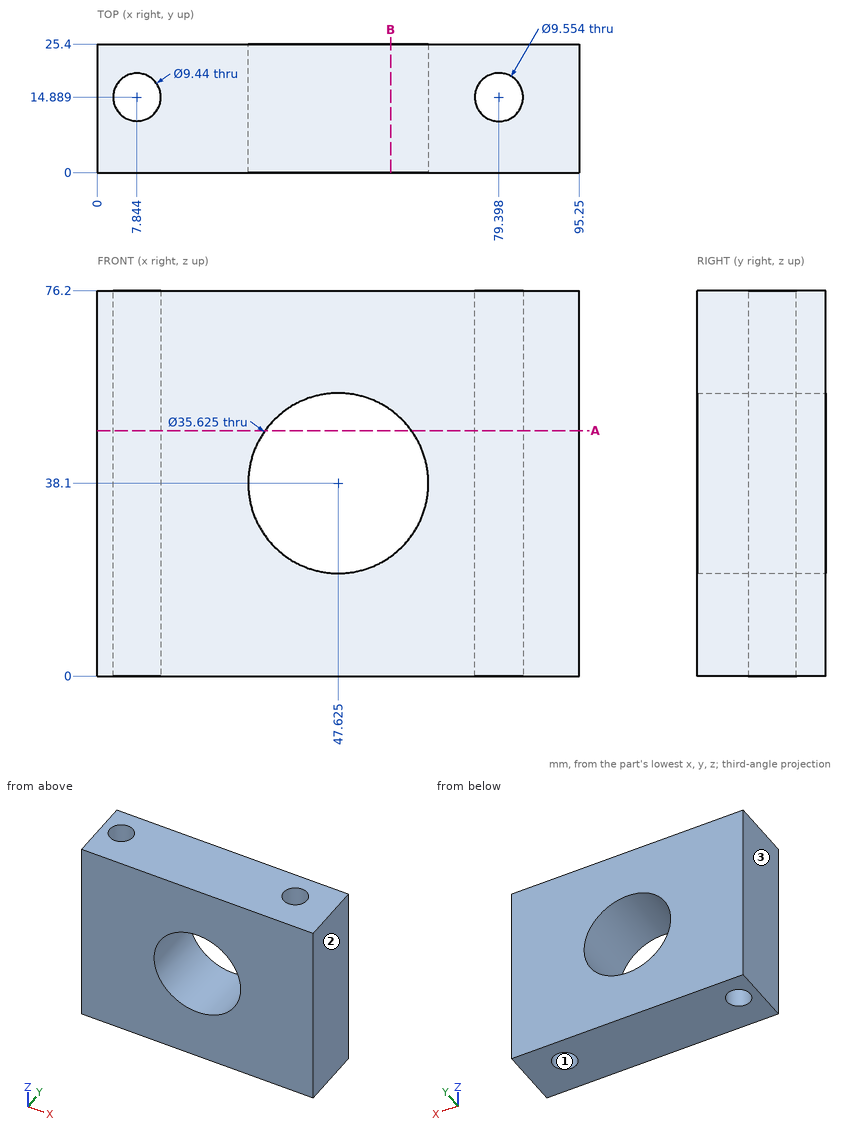
For this review, use the dimensioned drawing (mm, ordinates from the lowest corner) and the shaded views. Round coordinates to 2 decimals unless told otherwise and drop trailing zeros. Order: outer loops, then holes, each group sorted by start corner. A loop starts at its lowest first (then second) coordinate and runs counter-clockwise, first axis right, second up. Notation, with made-up numbers: (-5.5, 87) -> (45.5, 87) arc R33 ccw to (45.5, 120) -> close; hole circle Ø3 at (87.25, 34.5). An arc over 180 degrees is marked (long way). Write item = value, one per line. Start each with the question number.
Item 1: For line 1 along Z through (x, y) = (47, 14.5); line 2 along X through (y, z) = (3, 39.5); line 3 along Y through (x, z) = (9, 52) (1 decimal), list the stretches that pass through material, from the lowest coordinate up.
Item 2: Clearance check with flat-ended pins moving along their axes: pin 1 Ø1.5 at (y, z) = (19, 63.5) entering from -X; pin 2 Ø5.5 at (x, y) = (79.4, 14.89) entering from -Z. State where each tip first meets the part, or that it passes through.
Item 3: Mouldability with a two-part tool opening along X and no side actions: class the marked faces 1, 2 and 3 as released by +X, released by -X, zero draft, split by the parting line, or undercut.
Item 4: Consider section A-A on z = 48.5. Count the separate pieces of the cut face and the enclosed holes in it, plus the area to 3 significant figures.
Item 5: Consider section B-B on x = 58. Write out the cut boundary in (y, z), plus the area to 3 significant figures.
Conclusion:
q1.line_1 = 0 to 20.3, 55.9 to 76.2
q1.line_2 = 0 to 29.87, 65.38 to 95.25
q1.line_3 = 0 to 10.3, 19.5 to 25.4
q2.pin_1 = 0
q2.pin_2 = through
q3.face_1 = undercut
q3.face_2 = released by +X
q3.face_3 = released by -X
q4.separate_pieces = 2
q4.enclosed_holes = 2
q4.area = 1,540 mm2
q5.outline = (0, 0) -> (25.4, 0) -> (25.4, 23.62) -> (0, 23.62) -> close; (0, 52.58) -> (25.4, 52.58) -> (25.4, 76.2) -> (0, 76.2) -> close
q5.area = 1,200 mm2
